Geometry check sheet. Reference: the model listing, model coordinates, mm. A direction names the side the tool comes from. Coordinates: 2 decimals unless noted, no trailing zeros. Loops run counter-clockwise (first coordinate to the right, second up) from the corner with the lowest first, then second, coordinate; pieces in that order, holes last.
from build123d import *

# Parameters (mm, degrees)
BOSS_EXTRUDE1_DEPTH = 3.175
SKETCH2_W           = 3.175
SKETCH2_H           = 5
BOSS_EXTRUDE2_DEPTH = 3.175
CUT_EXTRUDE1_DEPTH  = 67.034660983


with BuildPart() as part:
    # Sketch1 → Boss-Extrude1 (new body)
    with BuildSketch(Plane.XY):
        with BuildLine():
            Line((39.415, -20), (39.415, 40))
            ThreePointArc((39.415, 40), (0, 12.507162886), (-39.415, 40))
            Line((-39.415, 40), (-39.415, -20))
            Line((-39.415, -20), (-3.785575219, -49.896637192))
            ThreePointArc((-3.785575219, -49.896637192), (-3.184040287, -50.243933548), (-2.5, -50.364548306))
            Line((-2.5, -50.364548306), (2.5, -50.364548306))
            ThreePointArc((2.5, -50.364548306), (3.184040287, -50.243933548), (3.785575219, -49.896637192))
            Line((3.785575219, -49.896637192), (39.415, -20))
        make_face()
    extrude(amount=BOSS_EXTRUDE1_DEPTH)

    # Sketch2 → Boss-Extrude2 (add)
    with BuildSketch(Plane.XY.offset(3.175)):
        with Locations((41.0025, -5)):
            Rectangle(SKETCH2_W, SKETCH2_H)
        with Locations((41.0025, 5)):
            Rectangle(SKETCH2_W, SKETCH2_H)
        with Locations((-41.0025, 5)):
            Rectangle(SKETCH2_W, SKETCH2_H)
        with Locations((-41.0025, -5)):
            Rectangle(SKETCH2_W, SKETCH2_H)
    extrude(amount=-BOSS_EXTRUDE2_DEPTH)

    # Sketch3 → Cut-Extrude1 (cut, through all)
    with BuildSketch(Plane.XY.offset(3.175)):
        Polygon((39.415, 1.5), (35.415, 1.5), (35.415, 3.05), (33.015, 3.05), (33.015, 1.5), (26.59, 1.5), (26.59, -1.5), (33.015, -1.5), (33.015, -3.05), (35.415, -3.05), (35.415, -1.5), (39.415, -1.5), align=None)
        Polygon((-39.415, -1.5), (-35.415, -1.5), (-35.415, -3.05), (-33.015, -3.05), (-33.015, -1.5), (-26.59, -1.5), (-26.59, 1.5), (-33.015, 1.5), (-33.015, 3.05), (-35.415, 3.05), (-35.415, 1.5), (-39.415, 1.5), align=None)
    extrude(amount=-CUT_EXTRUDE1_DEPTH, mode=Mode.SUBTRACT)


solid = part.part
1) Section check D-D on y = -42.5. Record the cut outline in (x, z) (3 decimals).
Data:
outline: (-12.601, 0) - (12.601, 0) - (12.601, 3.175) - (-12.601, 3.175) - close
2) Section check C-C on x = -5. Record the cut outline in (y, z) (3 decimals).
Data:
outline: (-48.878, 0) - (12.806, 0) - (12.806, 3.175) - (-48.878, 3.175) - close
3) Section check A-A on y = 27. Record the cut outline in (x, z) (3 decimals), and give its area (3 significant figures).
Data:
outline: (-39.415, 0) - (-31.739, 0) - (-31.739, 3.175) - (-39.415, 3.175) - close; (31.739, 0) - (39.415, 0) - (39.415, 3.175) - (31.739, 3.175) - close
area: 48.7 mm2
4) Depth check by flat-ended pin: pin 1 (0.7 mm diameter, centred on x = 34.5, z = 1, fed in from +Y); pin 2 (1 mm diameter, centred on x = 40.5, z = 2, fed in from +Y); pin 3 (1.6 mm diameter, centred on y = -14, z = 2.5, fed in from +X) (3 decimals). Enter the tip coordinate at first touch or a pass-through.
Data:
pin 1: stops at y = 31.07
pin 2: stops at y = 7.5
pin 3: stops at x = 39.415
5) Access from +Z, -Z, +X, -X, +Y, -Y to the whole of each face (thin tool, end or side, straight path). Record for faces 1 (the flat face through (-39.415, 24, 2)), 2 (the flat face through (-26.59, 0, 2)), 3 (the flat face through (41, 7.5, 2)), 4 (the flat face through (37, 1.5, 2)).
Data:
face 1: +Z, -Z, -X, +Y
face 2: +Z, -Z, -X
face 3: +Z, -Z, +X, +Y
face 4: +Z, -Z, +X
6) Material ranges on probe 1 along X at (y, z) = (2, 0.4) (3 decimals); probe 2 along X at (y, z) = (23, 2.1) (3 decimals); probe 3 along X at (y, z) = (28.5, 2.2) (3 decimals), recorded low to high.
Data:
probe 1: x = -39.415 to -35.415, -33.015 to 33.015, 35.415 to 39.415
probe 2: x = -39.415 to -27.772, 27.772 to 39.415
probe 3: x = -39.415 to -32.979, 32.979 to 39.415
7) Section check B-B on x = 37.5. Record the cut outline in (y, z) (3 decimals), and give its area (3 significant figures).
Data:
outline: (-21.607, 0) - (-1.5, 0) - (-1.5, 3.175) - (-21.607, 3.175) - close; (1.5, 0) - (35.593, 0) - (35.593, 3.175) - (1.5, 3.175) - close
area: 172 mm2
8) Mould release check, pull along X, two halves, no side actions. Record for faces 5 (the flat face through (-42.59, 5, 2)), 6 (the flat face through (39.415, -14, 2)), 7 (the cylindrical face through (0.716, 12.513, 1.565)): +X half, -X half, draft (parallel to the pull), parting line (faces both ways), or undercut.
Data:
face 5: -X half
face 6: +X half
face 7: undercut
